```python
from build123d import *

# Parameters (mm, degrees)
SKETCH_1_W      = 170
SKETCH_1_H      = 70
EXTRUDE_1_DEPTH = 35
EXTRUDE_START   = -35
EXTRUDE_2_DEPTH = 5


with BuildPart() as part:
    # Эскиз1 → Бобышка-Вытянуть1 (new body, symmetric)
    with BuildSketch(Plane.XY):
        Rectangle(SKETCH_1_W, SKETCH_1_H)
    extrude(amount=EXTRUDE_1_DEPTH, both=True)

    # Эскиз2 → Бобышка-Вытянуть2 (add, symmetric)
    with BuildSketch(Plane.XZ.offset(35).offset(EXTRUDE_START)):
        Polygon((33.713551402, 35), (-1.569013743, 35), (-1.526040465, 36.230593665), align=None)
    extrude(amount=EXTRUDE_2_DEPTH, both=True)


solid = part.part
```
For this review, take the finished solid that the model builds, in its own axes (mm). Round coordinates to 2 decimals unless told otherwise and drop trailing zeros. Write each loop counter-clockwise with the first axis right and the second up, starting at its lowest first coordinate (ties: lowest second). Pieces come first, ordered by that corner, then holes. Notation, with made-up numbers: (48, 61) -> (99, 61) arc R36 ccw to (99, 96) -> close; hole circle Ø8 at (71.25, -31). An arc over 180 degrees is marked (long way). Use one line per item in the form item = value.
Q1. To check wall thickness, follow probe 1 along Z at (x, y) = (-10, 17.5). State the ranges of the line that lie inside material, in increasing order. Write a range as from..to.
Resolved:
probe_1 = -35..35
Q2. Consider section B-B (y = 10). State the section outline as (x, z) points.
Resolved:
outline = (-85, -35) -> (85, -35) -> (85, 35) -> (-85, 35) -> close
Q3. Consider section A-A (x = 31.5). State the section outline as (y, z) points.
Resolved:
outline = (-35, -35) -> (35, -35) -> (35, 35) -> (5, 35) -> (5, 35.08) -> (-5, 35.08) -> (-5, 35) -> (-35, 35) -> close
Q4. Clearance check with flat-ended pins moving along their axes: pin 1 Ø5 at (x, y) = (29.5, 26) entering from +Z; pin 2 Ø0.6 at (x, z) = (15.5, 36) entering from -Y; pin 3 Ø0.6 at (x, z) = (24, 35.5) entering from +Y. State where each tip first meets the part, or that it passes through.
Resolved:
pin_1 = 35
pin_2 = through
pin_3 = 5
Q5. Consider section C-C (x = -37). State the section outline as (y, z) points, then the cut area to 3 significant figures.
Resolved:
outline = (-35, -35) -> (35, -35) -> (35, 35) -> (-35, 35) -> close
area = 4,900 mm²
